Source: CAD feature listing. Evaluate the final solid. Frame: model axes, mm. Face numbers are marked on the shaded views. A direction names the side the tool comes from. Coordinates: 2 decimals unless noted, no trailing zeros. Write each loop counter-clockwise with the first axis right and the second up, starting at its lowest first coordinate (ties: lowest second). Pieces come first, ordered by that corner, then holes. Notation, with made-up numbers: (-9, -11) - (37, -11) arc R20 ccw to (37, 23) - close; hole circle Ø10 at (68.25, -32.5). An arc over 180 degrees is marked (long way). One line per question, with ' | ' between items. Start each with the question number.
Q1. Access query for the marked faces 1, 2 and 3. Directions: +Z, -Z, +X, -X, +Y, -Y. A direction counts if a zero-diameter tool reaches every point of the face in a straight line with its end or side. Return the directions, or none.
Q2. Contact query for flat-ended pins moving along their axis: P1, Ø8, axis at x = 89, y = 1, coming from the +Z side; P2, Ø1, axis at x = 138.5, y = -6, coming from the -Z side; P3, Ø10, axis at y = 6.5, z = 35, coming from the +X side. Output: stop coordinate, or through.
Q3. Draft query along Z for the marked faces 4, 5 and 6. Return one class per face: +Z half, -Z half, draft (parallel to the pull), parting line (faces both ways), or undercut.
Q4. Cut plane D-D, the plane z = 13. Return loops of the section in (x, y), plus the area to 3 significant figures.
Q5. Cut plane C-C, the plane z = 28. Return loops of the section in (x, y).
Q6. Cut plane A-A, the plane y = 10. Return loops of the section in (x, z), plus the area to 3 significant figures.
Q7. Line query: line 1 (X direction, y = -18, z = 23.5); line 2 (X direction, y = 6, z = 25); line 3 (Z direction, x = 34, y = -15). Output: solid intervals per line, ascending.
Q8. Cut plane B-B, the plane x = 39. Return loops of the section in (y, z).
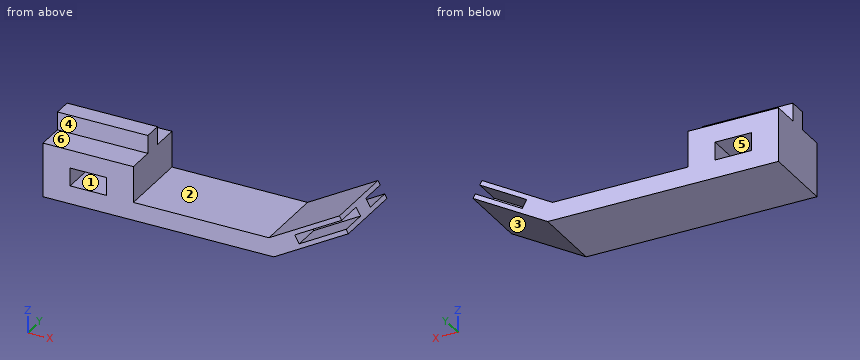
```python
from build123d import *

# Parameters (mm, degrees)
F0_W     = 20
F0_H     = 10
F1_DEPTH = 20
F0_W_2   = 50
F2_DEPTH = 5
F4_DEPTH = 15


with BuildPart() as f1:
    # F0 (on Front) → F1 (new body)
    with BuildSketch(Plane.XZ):
        Polygon((50, 30), (0, 30), (0, 0), (127.679492, 0), (168.971143, 23.839746), (163.971143, 32.5), (125, 10), (50, 10), align=None)
        with Locations((25, 15)):
            Rectangle(F0_W, F0_H, mode=Mode.SUBTRACT)
    extrude(amount=F1_DEPTH)

    # F0 (on Front) → F2 (join)
    with BuildSketch(Plane.XZ):
        with Locations((25, 35)):
            Rectangle(F0_W_2, F0_H)
    extrude(amount=F2_DEPTH)

    # F3 (on face) → F4 (cut)
    with BuildSketch(Plane.XZ.offset(20)):
        Polygon((167.721143, 26.004809), (165.221143, 30.334936), (139.240381, 15.334936), (141.740381, 11.004809), align=None)
    extrude(amount=-F4_DEPTH, mode=Mode.SUBTRACT)

    # F5: F1 across plane


with BuildPart() as f1_1:
    add(f1.part)
    add(f1.part.mirror(Plane.XZ))


solid = f1_1.part
```
Reply:
1) face 1: +Y, -Y | face 2: +Z, +Y, -Y | face 3: -Z, +X, +Y, -Y
2) P1: stops at z = 10 | P2: stops at z = 5.96 | P3: stops at x = 165.28
3) face 4: draft | face 5: undercut | face 6: +Z half
4) outline: (0, -20) - (15, -20) - (15, 20) - (0, 20) - close; (35, -20) - (50, -20) - (50, 20) - (35, 20) - close; (130.2, -20) - (140.59, -20) - (140.59, -5) - (145.2, -5) - (145.2, -20) - (150.2, -20) - (150.2, 20) - (145.2, 20) - (145.2, 5) - (140.59, 5) - (140.59, 20) - (130.2, 20) - close | area: 1,860 mm^2
5) outline: (0, -20) - (50, -20) - (50, 20) - (0, 20) - close; (156.18, -20) - (161.18, -20) - (161.18, -5) - (166.57, -5) - (166.57, 5) - (161.18, 5) - (161.18, 20) - (156.18, 20) - close
6) outline: (0, 0) - (127.68, 0) - (168.97, 23.84) - (167.72, 26) - (141.74, 11) - (139.24, 15.33) - (165.22, 30.33) - (163.97, 32.5) - (125, 10) - (50, 10) - (50, 30) - (0, 30) - close; hole (15, 10) - (35, 10) - (35, 20) - (15, 20) - close | area: 2,380 mm^2
7) line 1: x = 0 to 50, 148.38 to 153.38, 163.38 to 168.38 | line 2: x = 0 to 50, 150.98 to 155.98, 165.98 to 168.3 | line 3: z = 0 to 10, 20 to 30
8) outline: (-20, 0) - (20, 0) - (20, 30) - (5, 30) - (5, 40) - (-5, 40) - (-5, 30) - (-20, 30) - close
